Could you check a few things on this drawing? It's one solid part, dimensions in mm from its lowest x, y, z. Give positions to 0.01 mm unless a question says otherwise; leave off trailing zeros. Order: outer loops, then holes, each group sorted by start corner. A loop starts at its lowest first (then second) coordinate and runs counter-clockwise, first axis right, second up. Notation, with made-up numbers: M -11,-11 L 16,-11 A27 ccw 16,5 Z; hole C 4.5,79.5 d1. An arc over 180 degrees is marked long. One line per item, written item: value. Start each with the question number.
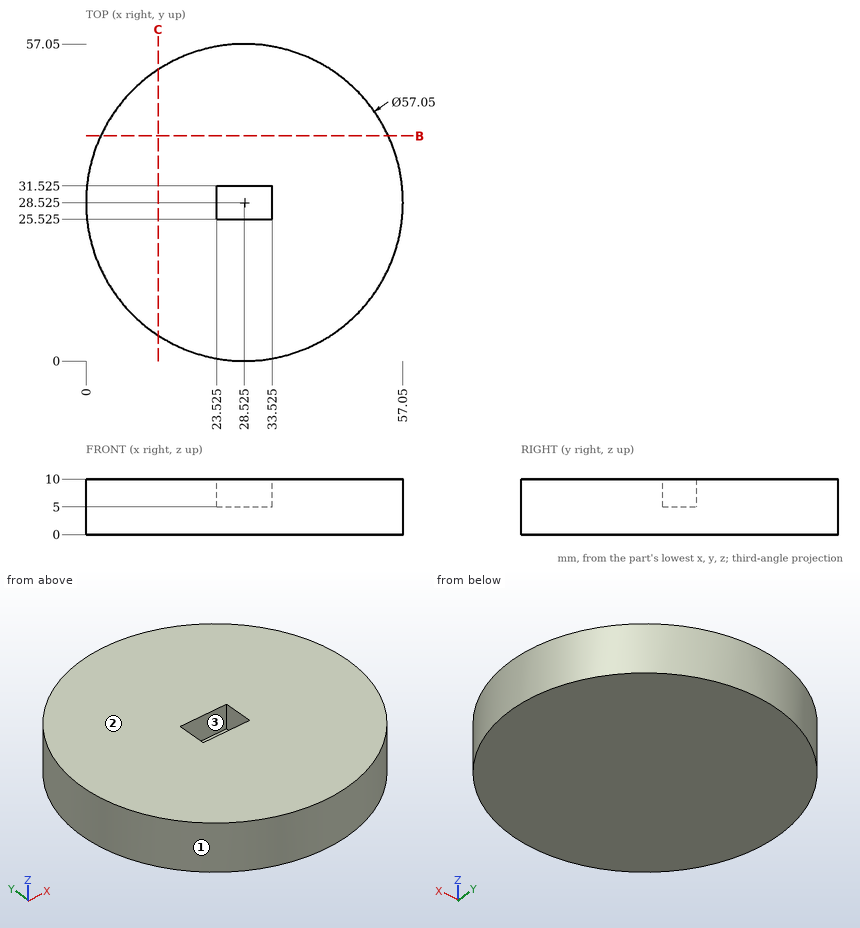
Item 1: Please list where these lines run through material, in increasing order: probe 1 along X at (y, z) = (31, 7.5) (1 decimal); probe 2 along X at (y, z) = (30, 6.75) (1 decimal); probe 3 along Y at (x, z) = (38, 7.75). Write a range as [from, to].
Item 2: I want a section at B-B on y = 40.5. Write out the boundary of the cut face in (x, z) (1 decimal), plus the area to 3 significant figures.
Item 3: We'd pull the mould along X, two halves only. Please class the marked faces 1, 2 and 3: +X half, -X half, draft (parallel to the pull), parting line (faces both ways), or undercut.
Item 4: I want a section at C-C on x = 13. Write out the boundary of the cut face in (y, z) (1 decimal).
Item 5: Will these pins go through, and if not, where does the flat tip stop? P1, Ø2, axis at x = 50, z = 8, coming from the -Y side (1 decimal); P2, Ø1, axis at x = 16.5, z = 7, coming from the -Y side; P3, Ø4, axis at x = 28, z = 8.5, coming from the -Y side.
Answer below:
1. probe 1: x = [0.1, 23.5], [33.5, 56.9]
1. probe 2: x = [0, 23.5], [33.5, 57]
1. probe 3: y = [1.62, 55.43]
2. outline: M 2.6,0 L 54.4,0 L 54.4,10 L 2.6,10 Z
2. area: 518 mm²
3. face 1: parting line
3. face 2: draft
3. face 3: undercut
4. outline: M 4.6,0 L 52.5,0 L 52.5,10 L 4.6,10 Z
5. P1: stops at y = 8.7
5. P2: stops at y = 2.43
5. P3: stops at y = 0
